from build123d import *

# Parameters (mm, degrees)
SKETCH1_W                = 77
SKETCH1_H                = 77
SKETCH1_W_2              = 14
SKETCH1_H_2              = 14
BOSS_EXTRUDE1_DEPTH      = 2
SKETCH2_R                = 1
CUT_EXTRUDE1_DEPTH       = 2
CHAMFER1_SIZE            = 1
CHAMFER1_OF_MIRROR1_SIZE = 1


with BuildPart() as part:
    # Sketch1 → Boss-Extrude1 (new body)
    with BuildSketch(Plane(origin=(0, 0, 0), x_dir=(1, 0, 0), z_dir=(0, 1, 0))):
        Rectangle(SKETCH1_W, SKETCH1_H)
        with Locations((-9.5, 28.5)):
            Rectangle(SKETCH1_W_2, SKETCH1_H_2, mode=Mode.SUBTRACT)
        with Locations((-28.5, 28.5)):
            Rectangle(SKETCH1_W_2, SKETCH1_H_2, mode=Mode.SUBTRACT)
        with Locations((9.5, 28.5)):
            Rectangle(SKETCH1_W_2, SKETCH1_H_2, mode=Mode.SUBTRACT)
        with Locations((28.5, 28.5)):
            Rectangle(SKETCH1_W_2, SKETCH1_H_2, mode=Mode.SUBTRACT)
        with Locations((-9.5, 9.5)):
            Rectangle(SKETCH1_W_2, SKETCH1_H_2, mode=Mode.SUBTRACT)
        with Locations((9.5, 9.5)):
            Rectangle(SKETCH1_W_2, SKETCH1_H_2, mode=Mode.SUBTRACT)
        with Locations((28.5, 9.5)):
            Rectangle(SKETCH1_W_2, SKETCH1_H_2, mode=Mode.SUBTRACT)
        with Locations((-9.5, -9.5)):
            Rectangle(SKETCH1_W_2, SKETCH1_H_2, mode=Mode.SUBTRACT)
        with Locations((9.5, -9.5)):
            Rectangle(SKETCH1_W_2, SKETCH1_H_2, mode=Mode.SUBTRACT)
        with Locations((28.5, -9.5)):
            Rectangle(SKETCH1_W_2, SKETCH1_H_2, mode=Mode.SUBTRACT)
        with Locations((-9.5, -28.5)):
            Rectangle(SKETCH1_W_2, SKETCH1_H_2, mode=Mode.SUBTRACT)
        with Locations((9.5, -28.5)):
            Rectangle(SKETCH1_W_2, SKETCH1_H_2, mode=Mode.SUBTRACT)
        with Locations((28.5, -28.5)):
            Rectangle(SKETCH1_W_2, SKETCH1_H_2, mode=Mode.SUBTRACT)
        with Locations((-28.5, 9.5)):
            Rectangle(SKETCH1_W_2, SKETCH1_H_2, mode=Mode.SUBTRACT)
        with Locations((-28.5, -9.5)):
            Rectangle(SKETCH1_W_2, SKETCH1_H_2, mode=Mode.SUBTRACT)
        with Locations((-28.5, -28.5)):
            Rectangle(SKETCH1_W_2, SKETCH1_H_2, mode=Mode.SUBTRACT)
    extrude(amount=BOSS_EXTRUDE1_DEPTH)

    # Sketch2 → Cut-Extrude1 (cut)
    with BuildSketch(Plane(origin=(0, 2, 0), x_dir=(1, 0, 0), z_dir=(0, 1, 0))):
        with Locations(Location((-19, 19, 0), (0, 0, 270))):
            Circle(SKETCH2_R)
        with Locations(Location((-28.5, -19, 0), (0, 0, 270))):
            Circle(SKETCH2_R)
    cut_extrude1 = extrude(amount=-CUT_EXTRUDE1_DEPTH, mode=Mode.SUBTRACT)

    # Chamfer1
    chamfer1_edges = [part.edges().sort_by_distance(p)[0] for p in [
        (-19, 2, -20),
        (-28.5, 2, 18),
    ]]
    chamfer(chamfer1_edges, length=CHAMFER1_SIZE)

    # Mirror1: Cut-Extrude1 across plane
    add(cut_extrude1.mirror(Plane(origin=(0, 0, 0), x_dir=(0, 0, 1), z_dir=(1, 0, 0))), mode=Mode.SUBTRACT)

    # Chamfer1 of Mirror1
    chamfer1_of_mirror1_edges = [part.edges().sort_by_distance(p)[0] for p in [
        (19, 2, -20),
        (28.5, 2, 18),
    ]]
    chamfer(chamfer1_of_mirror1_edges, length=CHAMFER1_OF_MIRROR1_SIZE)


solid = part.part
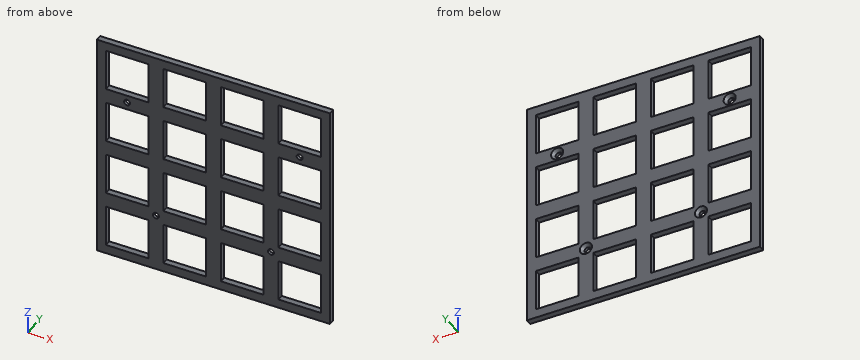
Read the model definition and answer for the solid it produces. Units are mm, in the model's axes. Round coordinates to 2 decimals unless told otherwise and drop trailing zeros. Write each loop counter-clockwise with the first axis right and the second up, starting at its lowest first coordinate (ties: lowest second). Pieces come first, ordered by that corner, then holes. Notation, with made-up numbers: (34, -6.5) - (42, -6.5) arc R20 cw to (42, -1.5) - close; hole circle Ø10 at (-30.5, -23). An arc over 180 degrees is marked (long way). One line per question, with ' | ' between items. Start each with the question number.
1. Section B-B (z = 19) is taken. Determine the outline of the cut face in (x, y), and give its area (3 significant figures).
2. Section D-D (y = 1.5) is taken. Give the number of separate pieces and of enclosed holes in the cut face, and give its area (3 significant figures).
3. Find the intervals of material crossed by probe 1 along X at (y, z) = (0.45, -19); probe 2 along Z at (x, y) = (24.5, 0.65); probe 3 along Z at (x, y) = (28.5, 0.75), in increasing order. Write a range as [from, to].
4. Section C-C (x = -28.5) is taken. Determine the outline of the cut face in (y, z), and give its area (3 significant figures).
5. Each of these flat-tipped pins is pushed along its axis until it touches: pin 1 (2.5 mm diameter, centred on x = -28.5, z = 19, fed in from +Y); pin 2 (2 mm diameter, centred on x = -12, z = -5, fed in from -Y). Where does it stop, or does it pass through?
6. Section A-A (x = -7.5) is taken. Determine the outline of the cut face in (y, z), and give its area (3 significant figures).
Filled in:
1) outline: (-38.5, 0) - (-29.5, 0) - (-29.5, 1) - (-30.5, 2) - (-38.5, 2) - close; (-27.5, 0) - (27.5, 0) - (27.5, 1) - (26.5, 2) - (-26.5, 2) - (-27.5, 1) - close; (29.5, 0) - (38.5, 0) - (38.5, 2) - (30.5, 2) - (29.5, 1) - close | area: 144 mm²
2) separate pieces: 1 | enclosed holes: 20 | area: 2,760 mm²
3) probe 1: [-38.5, -20], [-18, 18], [20, 38.5] | probe 2: [-38.5, -35.5], [-21.5, -16.5], [-2.5, 2.5], [16.5, 21.5], [35.5, 38.5] | probe 3: [-38.5, -35.5], [-21.5, -16.5], [-2.5, 2.5], [16.5, 18], [20, 21.5], [35.5, 38.5]
4) outline: (0, -38.5) - (2, -38.5) - (2, -35.5) - (0, -35.5) - close; (0, -21.5) - (2, -21.5) - (2, -16.5) - (0, -16.5) - close; (0, -2.5) - (2, -2.5) - (2, 2.5) - (0, 2.5) - close; (0, 16.5) - (2, 16.5) - (2, 17) - (1, 18) - (0, 18) - close; (0, 20) - (1, 20) - (2, 21) - (2, 21.5) - (0, 21.5) - close; (0, 35.5) - (2, 35.5) - (2, 38.5) - (0, 38.5) - close | area: 37.0 mm²
5) pin 1: y = 1.25 | pin 2: through
6) outline: (0, -38.5) - (2, -38.5) - (2, -35.5) - (0, -35.5) - close; (0, -21.5) - (2, -21.5) - (2, -16.5) - (0, -16.5) - close; (0, -2.5) - (2, -2.5) - (2, 2.5) - (0, 2.5) - close; (0, 16.5) - (2, 16.5) - (2, 21.5) - (0, 21.5) - close; (0, 35.5) - (2, 35.5) - (2, 38.5) - (0, 38.5) - close | area: 42.0 mm²
